Autodesk Inventor part; units mm, degrees
ref_plane "YZ Plane" through (0, 0, 0) normal (1, 0, 0) x (0, 1, 0)
ref_plane "XZ Plane" through (0, 0, 0) normal (0, 1, 0) x (-1, 0, 0)
ref_plane "XY Plane" through (0, 0, 0) normal (0, 0, 1) x (1, 0, 0)
sketch "スケッチ1" plane through (0, 0, 0) normal (0, 0, 1) x (1, 0, 0)
  line L0 (4.5, 0.9036) -> (4.5, -2.75)
  line L1 (4.5, -2.75) -> (2, -2.75)
  line L2 (0, 2.75) -> (0, -2.75)
  line L3 (3.9, 1.25) -> (4.5, 0.9036)
  line L4 (2, -2.75) -> (2, 2.75)
  line L5 (2, 2.75) -> (3.7, 2.75)
  line L6 (3.9, 1.25) -> (3.7, 1.25)
  line L7 (3.7, 1.25) -> (3.7, 2.75)
  point P0 (0, 0)
  dimension "d3" = 4.5
  dimension "d14" = 2.75
  dimension "d15" = 5.5
  dimension "d16" = 2.75
  dimension "d17" = 5.5
  dimension "d18" = 2.5
  dimension "d20" = 120
  dimension "d28" = 1.7
  dimension "d29" = 1.5
  dimension "d30" = 0.2
revolve "回転1" add sketch "スケッチ1" angle 360 about axis through (0, 2.75, 0) along (0, -1, 0)
sketch "スケッチ3" plane through (0, -2.75, 0) normal (0, -1, 0) x (1, 0, 0)
  circle A0 centre (0, 0) radius 2
  circle A1 centre (0, 0) radius 4.5
  line L0 (0, 4.5) -> (3.8971, 2.25)
  line L1 (3.8971, 2.25) -> (3.8971, -2.25)
  line L2 (3.8971, -2.25) -> (0, -4.5)
  line L3 (0, -4.5) -> (-3.8971, -2.25)
  line L4 (-3.8971, -2.25) -> (-3.8971, 2.25)
  line L5 (-3.8971, 2.25) -> (0, 4.5)
  dimension "d23" = 2.25
extrude "押し出し2" cut sketch "スケッチ3" against normal blind 5.5 contours L1 L2 L3 L4 L5 L0 keep common part
fillet "フィレット1" radius 0.5 2 edges at (-3.7, 2.75, 0) (-2, -2.75, 0)
sketch "スケッチ4" plane through (0, 2.75, 0) normal (0, 1, 0) x (1, 0, 0)
  circle A0 centre (0, 0) radius 2
  circle A1 centre (0, 0) radius 3.2
  circle A2 centre (0, 0) radius 2.5
  dimension "d32" = 5
extrude "押し出し3" cut sketch "スケッチ4" against normal blind 0.2 contours A2
fillet "フィレット2" radius 0.1 2 edges at (-2, 2.55, 0) (-2.5, 2.75, 0)
thread "ねじ3"
properties material "ステンレス鋼"
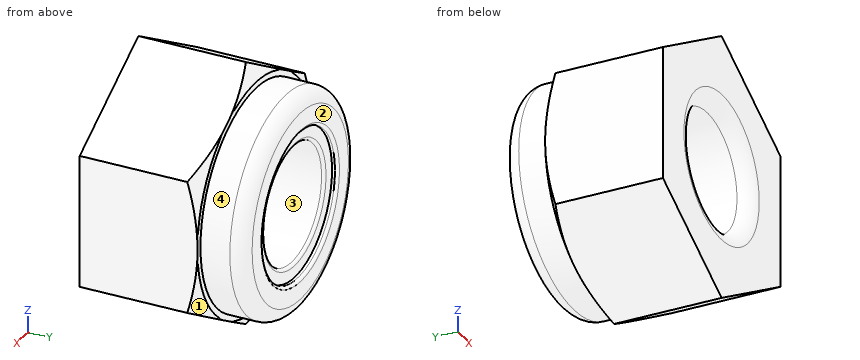
Verification items for the finished model (mm, model axes). Face numbers are marked on the shaded views. Coordinates: 2 decimals unless noted, no trailing zeros. Order: outer loops, then holes, each group sorted by start corner. A loop starts at its lowest first (then second) coordinate and runs counter-clockwise, first axis right, second up. Notation, with made-up numbers: (16.5, 5) -> (56.5, 5) arc R19 cw to (56.5, 10) -> close; hole circle Ø8 at (60.25, 49). An arc over 180 degrees is marked (long way). Use CSV: the item, a comma, the result in double quotes. Start each with the question number.
Q1. Section check C-C, the plane y = 1.4. Record the cut outline in (x, z), and give its area (3 significant figures).
Q2. Draft check along X on the marked faces 1, 2, 3 and 4. Enter one of: +X half, -X half, draft (parallel to the pull), parting line (faces both ways), or undercut.
Q3. Thickness scan on line 1 along X through (y, z) = (-0.9, 0); line 2 along Z through (x, y) = (0, 1.4); line 3 along Z through (x, y) = (0, 2.65). Record the ranges inside material, lowest first.
Q4. Section check A-A, the plane z = 0. Record the cut outline in (x, y), and give its area (3 significant figures).
Q5. Section check B-B, the plane y = -0.2. Record the cut outline in (x, z), and give its area (3 significant figures).
Q6. Depth check by flat-ended pin: P1, Ø3, axis at x = -1, y = -0.5, coming from the -Z side; P2, Ø3, axis at y = -1, z = 2.5, coming from the -X side; P3, Ø2.5, axis at x = -0.5, z = -0.5, coming from the +Y side. Enter the tip coordinate at first touch or a pass-through.
Returned:
1,outline,"circle Ø7.4 at (0, 0); hole circle Ø4 at (0, 0)"
1,area,"30.4 mm^2"
2,face 1,"+X half"
2,face 2,"draft"
2,face 3,"undercut"
2,face 4,"parting line"
3,line 1,"x = -3.9 to -2, 2 to 3.9"
3,line 2,"z = -3.7 to -2, 2 to 3.7"
3,line 3,"z = -3.5 to -2.5, 2.5 to 3.5"
4,outline,"(-3.9, -2.75) -> (-2.5, -2.75) arc R0.5 ccw to (-2, -2.25) -> (-2, 2.45) arc R0.1 ccw to (-2.1, 2.55) -> (-2.5, 2.55) -> (-2.5, 2.65) arc R0.1 ccw to (-2.6, 2.75) -> (-3.2, 2.75) arc R0.5 ccw to (-3.7, 2.25) -> (-3.7, 1.25) -> (-3.9, 1.25) -> close; (2, -2.25) arc R0.5 ccw to (2.5, -2.75) -> (3.9, -2.75) -> (3.9, 1.25) -> (3.7, 1.25) -> (3.7, 2.25) arc R0.5 ccw to (3.2, 2.75) -> (2.6, 2.75) arc R0.1 ccw to (2.5, 2.65) -> (2.5, 2.55) -> (2.1, 2.55) arc R0.1 ccw to (2, 2.45) -> close"
4,area,"19.9 mm^2"
5,outline,"(-3.9, -2.25) -> (0, -4.5) -> (3.9, -2.25) -> (3.9, 2.25) -> (0, 4.5) -> (-3.9, 2.25) -> close; hole circle Ø4 at (0, 0)"
5,area,"40.0 mm^2"
6,P1,"stops at z = -4.5"
6,P2,"stops at x = -3.9"
6,P3,"passes through"
